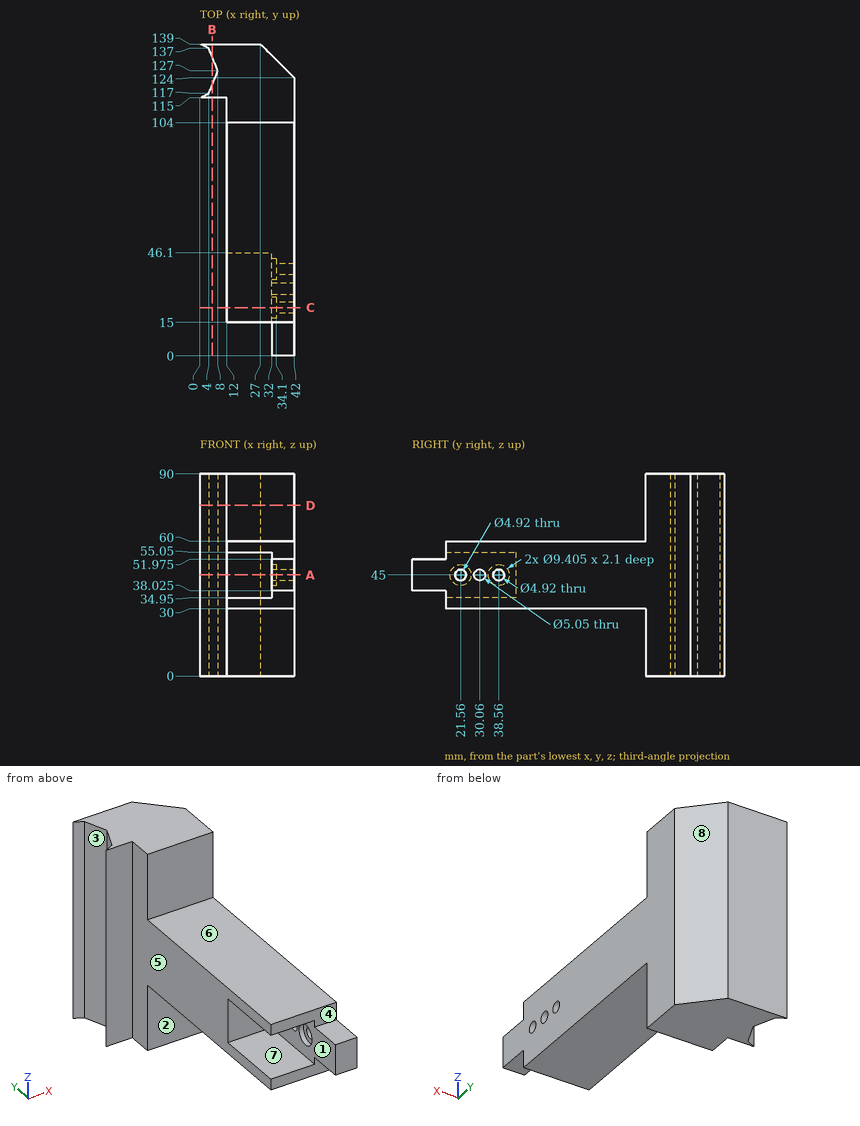
The figure shows three views and two pictorial views of one solid part (mm, origin at its lowest corner). Answer the questions. A direction names the side the tool comes from. Round coordinates to 2 decimals unless told otherwise and drop trailing zeros. Order: outer loops, then holes, each group sorted by start corner. A loop starts at its lowest first (then second) coordinate and runs counter-clockwise, first axis right, second up.
Q1. Find the intervals of material crossed by line 1 along Y through (x, z) = (40.25, 45) (3 decimals); line 2 along Z through (x, y) = (33, 21); line 3 along Z through (x, y) = (23.5, 16), in increasing order.
Solution:
line 1: y = 0 to 19.1, 24.02 to 27.535, 32.585 to 36.1, 41.02 to 125.75
line 2: z = 30 to 40.33, 49.67 to 60
line 3: z = 30 to 34.95, 55.05 to 60
Q2. A cutting plane is placed at A-A, the plane z = 45. Count the separate pieces of the cut face and the enclosed holes in it, then the cut area to 3 significant figures.
Solution:
separate pieces: 4
enclosed holes: 0
area: 3,130 mm2
Q3. A cutting plane is placed at B-B, the plane x = 5.5. Determine the outline of the cut face in (y, z), then the cut area to 4 significant figures.
Solution:
outline: (115, 0) - (120.75, 0) - (120.75, 90) - (115, 90) - close; (133.25, 0) - (139, 0) - (139, 90) - (133.25, 90) - close
area: 1,035 mm2
Q4. A cutting plane is placed at C-C, the plane y = 21.56. Determine the outline of the cut face in (x, z).
Solution:
outline: (12, 30) - (42, 30) - (42, 42.54) - (34.1, 42.54) - (34.1, 40.3) - (32, 40.3) - (32, 34.95) - (12, 34.95) - close; (12, 55.05) - (32, 55.05) - (32, 49.7) - (34.1, 49.7) - (34.1, 47.46) - (42, 47.46) - (42, 60) - (12, 60) - close
Q5. The mould has two halves that part along Z. Classify the marked faces 6, 7 and 8: pulls with the +Z half, pulls with the -Z half, needs draft (parallel to the pull), parting line crosses it, or undercut.
Solution:
face 6: pulls with the +Z half
face 7: undercut
face 8: needs draft
Q6. A tool of negligible diameter and unlimited length cuts with its end or side. For the marked faces 1, 2, 3, 4 and 5, from which of +Z, -Z, +X, -X, +Y, -Y can it reach the whole face along a straight path? Write none if from no direction.
Solution:
face 1: -X, -Y
face 2: -Z, +X, -X, -Y
face 3: +Z, -Z, -X
face 4: +Z, +X, -X, -Y
face 5: +Z, -Z, -X, -Y
Q7. Given pin 1 Ø5 at (x, z) = (25.5, 20) entering from -Y; pin 2 Ø2.5 at (x, z) = (25.5, 32.5) entering from -Y; pin 3 Ø10 at (x, y) = (23, 34) entering from +Z; pin 4 Ø3 at (y, z) = (22, 45) entering from -X, each flat-ended and moving along its own axis, determine where each tip first touches the part or whether it passes through.
Solution:
pin 1: stops at y = 104
pin 2: stops at y = 15
pin 3: stops at z = 60
pin 4: passes through
Q8. A cutting plane is placed at D-D, the plane z = 76. Determine the outline of the cut face in (x, y).
Solution:
outline: (0, 115) - (12, 115) - (12, 104) - (42, 104) - (42, 124) - (27, 139) - (0, 139) - (4, 137) - (8, 127) - (4, 117) - close
